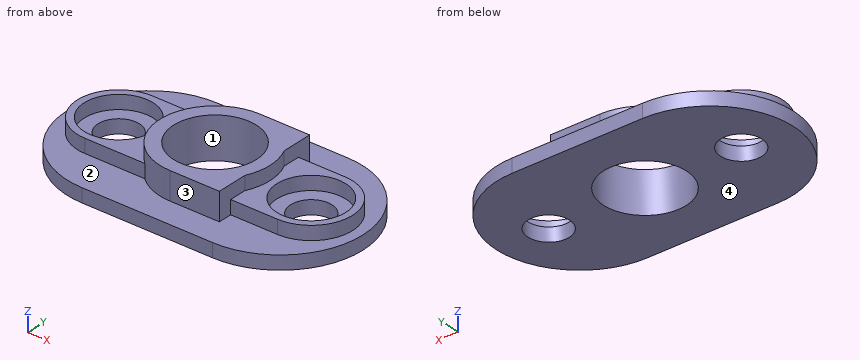
```python
from build123d import *

# Parameters (mm, degrees)
EXTRUSION1_DEPTH        = 2
EXTRUSION4_DEPTH        = 2
EXTRUSION5_DEPTH        = 4
ESQUISSE3_R             = 6
ENL_V_MAT_EXTRU_1_DEPTH = 5
ESQUISSE5_R             = 3
ENL_V_MAT_EXTRU_2_DEPTH = 5
ESQUISSE6_R             = 5
ENL_V_MAT_EXTRU_3_DEPTH = 2


with BuildPart() as part:
    # Esquisse1 → Extrusion1 (new body)
    with BuildSketch(Plane.XY):
        with BuildLine():
            Line((-57.049073, 33.907042), (-38.049073, 33.907042))
            ThreePointArc((-38.049073, 33.907042), (-26.049073, 21.907042), (-38.049073, 9.907042))
            Line((-38.049073, 9.907042), (-57.049073, 9.907042))
            ThreePointArc((-57.049073, 9.907042), (-69.049073, 21.907042), (-57.049073, 33.907042))
        make_face()
    extrude(amount=EXTRUSION1_DEPTH)

    # Esquisse2 → Extrusion4 (add)
    with BuildSketch(Plane.XY.offset(2)):
        with BuildLine():
            Line((-61.549073, 27.907042), (-33.549073, 27.907042))
            ThreePointArc((-33.549073, 27.907042), (-27.549073, 21.907042), (-33.549073, 15.907042))
            Line((-33.549073, 15.907042), (-61.549073, 15.907042))
            ThreePointArc((-61.549073, 15.907042), (-67.549073, 21.907042), (-61.549073, 27.907042))
        make_face()
    extrude(amount=EXTRUSION4_DEPTH)

    # Esquisse4 → Extrusion5 (add)
    with BuildSketch(Plane.XY.offset(2)):
        with BuildLine():
            Line((-47.549305, 29.907042), (-40.349305, 29.907042))
            Line((-40.349305, 29.907042), (-40.349305, 25.394161155))
            ThreePointArc((-40.349305, 25.394161155), (-39.549305, 21.907042), (-40.349305, 18.419922845))
            Line((-40.349305, 18.419922845), (-40.349305, 13.907042))
            Line((-40.349305, 13.907042), (-47.549305, 13.907042))
            ThreePointArc((-47.549305, 13.907042), (-55.549305, 21.907042), (-47.549305, 29.907042))
        make_face()
    extrude(amount=EXTRUSION5_DEPTH)

    # Esquisse3 → Enlèv. mat.-Extru.1 (cut, symmetric)
    with BuildSketch(Plane.XY.offset(4)):
        with Locations((-47.549073, 21.907042)):
            Circle(ESQUISSE3_R)
    extrude(amount=ENL_V_MAT_EXTRU_1_DEPTH, both=True, mode=Mode.SUBTRACT)

    # Esquisse5 → Enlèv. mat.-Extru.2 (cut, through all)
    with BuildSketch(Plane.XY.offset(4)):
        with Locations((-61.549073, 21.907042)):
            Circle(ESQUISSE5_R)
        with Locations((-33.549073, 21.907042)):
            Circle(ESQUISSE5_R)
    extrude(amount=-ENL_V_MAT_EXTRU_2_DEPTH, mode=Mode.SUBTRACT)

    # Esquisse6 → Enlèv. mat.-Extru.3 (cut)
    with BuildSketch(Plane.XY.offset(4)):
        with Locations((-61.549073, 21.907042)):
            Circle(ESQUISSE6_R)
        with Locations((-33.549073, 21.907042)):
            Circle(ESQUISSE6_R)
    extrude(amount=-ENL_V_MAT_EXTRU_3_DEPTH, mode=Mode.SUBTRACT)


solid = part.part
```
Work out the finished part from the listing and answer in its coordinate system (mm). Face numbers are marked on the shaded views. A direction names the side the tool comes from. Give positions to 0.01 mm unless a question says otherwise; leave off trailing zeros. Loops run counter-clockwise (first coordinate to the right, second up) from the corner with the lowest first, then second, coordinate; pieces in that order, holes last. Notation, with made-up numbers: (32.25, 47.25) -> (82.25, 47.25) arc R27 cw to (82.25, 68.25) -> close; hole circle Ø5 at (6.25, 64). An arc over 180 degrees is marked (long way). One line per question, with ' | ' between items. Start each with the question number.
1) Section C-C, the plane x = -48.5 is taken. Determine the outline of the cut face in (y, z).
2) Section B-B, the plane x = -41 is taken. Determine the outline of the cut face in (y, z).
3) Determine the mould class of the marked faces 1 and 2 for opening direction X: +X half, -X half, draft (parallel to the pull), parting line (faces both ways), or undercut.
4) Section A-A, the plane y = 24.5 is taken. State how many separate pieces and enclosed holes the cut face has, then the cut area to 3 significant figures.
5) For the marked faces 3 and 4, determine the directions among +Z, -Z, +X, -X, +Y, -Y from which every point of the face is accessible in a straight line to the end or side of a thin tool.
6) Section D-D, the plane y = 27.5 is taken. Determine the outline of the cut face in (x, z), then the cut area to 3 significant figures.
7) Straight lines are drawn through the part: L1, parallel to X at y = 21.25, z = 2.9; L2, parallel to Z at x = -56.5, y = 25.75; L3, parallel to Z at x = -64, y = 23.75. For each, find the intervals that lie inside material, in ascending order.
8) Each of these flat-tipped pins is pushed along its axis until it touches: pin 1 (3 mm diameter, centred on x = -33.5, y = 23, fed in from +Z); pin 2 (1.6 mm diameter, centred on x = -35.5, z = 3, fed in from +Y); pin 3 (1 mm diameter, centred on x = -39.5, y = 13, fed in from -Z); pin 4 (1.5 mm diameter, centred on y = 22, z = 4, fed in from -X). Where does it stop, or does it pass through?
Resolved:
1) outline: (9.91, 0) -> (15.98, 0) -> (15.98, 6) -> (13.96, 6) -> (13.96, 2) -> (9.91, 2) -> close; (27.83, 0) -> (33.91, 0) -> (33.91, 2) -> (29.85, 2) -> (29.85, 6) -> (27.83, 6) -> close
2) outline: (9.91, 0) -> (33.91, 0) -> (33.91, 2) -> (29.91, 2) -> (29.91, 6) -> (13.91, 6) -> (13.91, 2) -> (9.91, 2) -> close
3) face 1: undercut | face 2: draft
4) separate pieces: 4 | enclosed holes: 0 | area: 81.6 mm2
5) face 3: +Z, +X, -X, -Y | face 4: -Z, +X, -X, +Y, -Y
6) outline: (-67.67, 0) -> (-49.72, 0) -> (-49.72, 6) -> (-53.27, 6) -> (-53.27, 4) -> (-63.72, 4) -> (-63.72, 2) -> (-67.67, 2) -> close; (-45.38, 0) -> (-27.43, 0) -> (-27.43, 2) -> (-31.38, 2) -> (-31.38, 4) -> (-40.35, 4) -> (-40.35, 6) -> (-45.38, 6) -> close | area: 145 mm2
7) L1: -67.51 to -66.51, -56.59 to -53.51, -41.59 to -38.51, -28.59 to -27.59 | L2: 0 to 4 | L3: 0 to 2
8) pin 1: through | pin 2: y = 27.91 | pin 3: z = 0 | pin 4: x = -67.55
